Design review of the part built by this model. Coordinates are the model's own, in mm. A direction names the side the tool comes from. Give positions to 0.01 mm unless a question says otherwise; leave off trailing zeros. Loops run counter-clockwise (first coordinate to the right, second up) from the corner with the lowest first, then second, coordinate; pieces in that order, holes last. Notation, with made-up numbers: (-36.5, -36) -> (12.5, -36) arc R13 cw to (12.5, -22) -> close; hole circle Ø5 at (-37, -14.75). An arc over 180 degrees is marked (long way). Answer as CSV lines item,"result".
from build123d import *

# Parameters (mm, degrees)
ESBO_O2_W = 6
ESBO_O2_H = 2


with BuildPart() as part:
    # Varredura1: sweep along a path in Esboço1
    with BuildLine(Plane.XY) as varredura1_path:
        Line((-60.462858141, 17.215577733), (47.330289745, 36.890523713))
        ThreePointArc((47.330289745, 36.890523713), (91.563733155, 0), (47.330289745, -36.890523713))
        Line((47.330289745, -36.890523713), (-60.462858141, -17.215577733))
        ThreePointArc((-60.462858141, -17.215577733), (-74.82058455, 0), (-60.462858141, 17.215577733))
    # Esboço2 → Varredura1 (sweep)
    with BuildSketch(Plane(origin=(-60.462858141, 17.215577733, 0), x_dir=(0, 0, -1), z_dir=(0.9837472990234445, 0.17955849092726803, 0))):
        Rectangle(ESBO_O2_W, ESBO_O2_H)
    sweep(path=varredura1_path.line)


solid = part.part
Q1. The part is to be moulded in two halves that separate along X. For faces 1 (the cylindrical face through (-75.817, -0.36, 0.042)), 2 (the flat face through (4, 29, 3)), 3 (the flat face through (-7.14, -25.93, 0.04)), say which applies: pulls with the +X half, pulls with the -X half, needs draft (parallel to the pull), parting line crosses it, or undercut.
Filled sheet:
face 1,"pulls with the -X half"
face 2,"needs draft"
face 3,"undercut"
Q2. Clearance check with flat-ended pins moving along their axes: pin 1 Ø3 at (y, z) = (3, -1.5) entering from +X; pin 2 Ø1 at (y, z) = (6.5, 0.5) entering from +X. State where each tip first meets the part, or that it passes through.
Filled sheet:
pin 1,"stops at x = 92.53"
pin 2,"stops at x = 92.09"
Q3. We need section C-C, the plane x = 78. State the section outline as (y, z) points.
Filled sheet:
outline,"(-30.15, -3) -> (-27.56, -3) -> (-27.56, 3) -> (-30.15, 3) -> close; (27.56, -3) -> (30.15, -3) -> (30.15, 3) -> (27.56, 3) -> close"
Q4. To check wall thickness, follow probe 1 along Y at (x, z) = (54.5, 1); probe 2 along X at (y, z) = (-1, -0.5); probe 3 along X at (y, z) = (0, 1). State the ranges of each line that lie inside material, in increasing order. Write a range as from..to.
Filled sheet:
probe 1,"y = -38.5..-36.5, 36.5..38.5"
probe 2,"x = -75.79..-73.79, 90.55..92.55"
probe 3,"x = -75.82..-73.82, 90.56..92.56"
Q5. We need section B-B, the plane y = 22. State the section outline as (x, z) points, and give its area (3 significant figures).
Filled sheet:
outline,"(-39.82, -3) -> (-28.68, -3) -> (-28.68, 3) -> (-39.82, 3) -> close; (83.19, -3) -> (85.66, -3) -> (85.66, 3) -> (83.19, 3) -> close"
area,"81.7 mm^2"
Q6. We need section A-A, the plane z = -1.75. State the section outline as (x, y) points, and give its area (3 significant figures).
Filled sheet:
outline,"(-60.64, -18.2) -> (47.15, -37.87) arc R38.5 ccw (long way) to (47.15, 37.87) -> (-60.64, 18.2) arc R18.5 ccw to start; hole (-60.28, -16.23) -> (47.51, -35.91) arc R36.5 ccw (long way) to (47.51, 35.91) -> (-60.28, 16.23) arc R16.5 ccw to start"
area,"798 mm^2"
Q7. For faces 4 (the cylindrical face through (-73.817, -0.321, -0.042)), 5 (the flat face through (-7.5, -27.9, 0)), list the 3-axis set-ups (+Z, -Z, +X, -X, +Y, -Y) from which the entire face can be reached by the end or side of a thin tool; tool diameter is ignored.
Filled sheet:
face 4,"+Z, -Z"
face 5,"+Z, -Z, -X, -Y"
